```python
from build123d import *

# Parameters (mm, degrees)
BASE_FLANGE1_DEPTH                   = 3.175
EDGE_FLANGE1_DEPTH                   = 528.215976366
EDGE_FLANGE1_BEND_DEPTH              = 457.2
EDGE_FLANGE1_BEND_2_DEPTH            = 457.2
F_17_64_0_26563_DIAMETER_HOLE1_D     = 6.747002
F_17_64_0_26563_DIAMETER_HOLE1_DEPTH = 3.175
F_17_64_0_26563_DIAMETER_HOLE1_TIP   = 2.027003899
F_17_64_0_26563_DIAMETER_HOLE2_D     = 6.747002
F_17_64_0_26563_DIAMETER_HOLE2_DEPTH = 3.175
F_17_64_0_26563_DIAMETER_HOLE2_TIP   = 2.027003899
FILLET1_R                            = 3.175
F_17_64_0_26563_DIAMETER_HOLE3_D     = 6.747002
F_17_64_0_26563_DIAMETER_HOLE3_DEPTH = 3.175
F_17_64_0_26563_DIAMETER_HOLE3_TIP   = 2.027003899
F_17_64_0_26563_DIAMETER_HOLE4_D     = 6.747002


# Sheet-metal steps are written as plain solids
with BuildPart() as part:
    # Sketch1 → Base-Flange1 (new body)
    with BuildSketch(Plane(origin=(0, 0, 0), x_dir=(0, 0, -1), z_dir=(1, 0, 0))):
        Polygon((0, 12.7), (0, 469.9), (-11.934096284, 478.25634418), (-441.561562507, 321.884734651), (-443.092427829, 310.256658089), (-10.403230962, 7.284420742), align=None)
    extrude(amount=-BASE_FLANGE1_DEPTH)

    # Edge-Flange1 section (across the edge) → Edge-Flange1 (add)
    with BuildSketch(Plane(origin=(-3.175, 4.683613001, 12.224336148), x_dir=(-3.4914813388431334e-15, 0.819152044288993, -0.5735764363510446), z_dir=(0, 0.5735764363510446, 0.819152044288993))):
        with BuildLine():
            Line((-3.175, 3.175), (-3.175, 41.275))
            Line((-3.175, 41.275), (0, 41.275))
            Line((0, 41.275), (0, 3.175))
            ThreePointArc((0, 3.175), (0.92993597, 0.92993597), (3.175, 0))
            Line((3.175, 0), (3.175, -3.175))
            ThreePointArc((3.175, -3.175), (-1.315128061, -1.315128061), (-3.175, 3.175))
        make_face()
    extrude(amount=EDGE_FLANGE1_DEPTH)

    # Edge-Flange1 section 2 (across the edge) → Edge-Flange1 bend (add)
    with BuildSketch(Plane(origin=(-3.175, 469.9, -3.175), x_dir=(0, 0, 1), z_dir=(0, -1, 0))):
        with BuildLine():
            Line((-3.175, 3.175), (-3.175, 41.275))
            Line((-3.175, 41.275), (0, 41.275))
            Line((0, 41.275), (0, 3.175))
            ThreePointArc((0, 3.175), (0.92993597, 0.92993597), (3.175, 0))
            Line((3.175, 0), (3.175, -3.175))
            ThreePointArc((3.175, -3.175), (-1.315128061, -1.315128061), (-3.175, 3.175))
        make_face()
    extrude(amount=EDGE_FLANGE1_BEND_DEPTH)

    # Edge-Flange1 section 3 (across the edge) → Edge-Flange1 bend 2 (add)
    with BuildSketch(Plane(origin=(-3.175, 324.868258722, 442.647476462), x_dir=(-3.4914813388431334e-15, -0.9396926207859071, -0.3420201433256725), z_dir=(0, 0.3420201433256725, -0.9396926207859071))):
        with BuildLine():
            Line((-3.175, 3.175), (-3.175, 41.275))
            Line((-3.175, 41.275), (0, 41.275))
            Line((0, 41.275), (0, 3.175))
            ThreePointArc((0, 3.175), (0.92993597, 0.92993597), (3.175, 0))
            Line((3.175, 0), (3.175, -3.175))
            ThreePointArc((3.175, -3.175), (-1.315128061, -1.315128061), (-3.175, 3.175))
        make_face()
    extrude(amount=EDGE_FLANGE1_BEND_2_DEPTH)

    # 17/64 (0.26563) Diameter Hole1
    with Locations(Plane(origin=(0, 0, -6.35), x_dir=(-1, 0, 0), z_dir=(0, 0, -1))):
        with Locations((22.225, 390.525), (22.225, 31.75)):
            Hole(F_17_64_0_26563_DIAMETER_HOLE1_D / 2, depth=F_17_64_0_26563_DIAMETER_HOLE1_DEPTH)
            with Locations((0, 0, -(F_17_64_0_26563_DIAMETER_HOLE1_DEPTH + F_17_64_0_26563_DIAMETER_HOLE1_TIP / 2))):  # 118° drill point
                Cone(0, F_17_64_0_26563_DIAMETER_HOLE1_D / 2, F_17_64_0_26563_DIAMETER_HOLE1_TIP, mode=Mode.SUBTRACT)

    # 17/64 (0.26563) Diameter Hole2
    with Locations(Plane(origin=(0, 432.113572267, 157.276478127), x_dir=(1, 0, 0), z_dir=(3.4475760670445246e-15, 0.939692620785907, 0.3420201433256725))):
        with Locations((-22.225, 72.983921169), (-22.225, -285.791078831)):
            Hole(F_17_64_0_26563_DIAMETER_HOLE2_D / 2, depth=F_17_64_0_26563_DIAMETER_HOLE2_DEPTH)
            with Locations((0, 0, -(F_17_64_0_26563_DIAMETER_HOLE2_DEPTH + F_17_64_0_26563_DIAMETER_HOLE2_TIP / 2))):  # 118° drill point
                Cone(0, F_17_64_0_26563_DIAMETER_HOLE2_D / 2, F_17_64_0_26563_DIAMETER_HOLE2_TIP, mode=Mode.SUBTRACT)

    # Fillet1
    fillet1_edges = [part.edges().sort_by_distance(p)[0] for p in [
        (-44.45, 3.383209131, 13.134888741),
        (-44.45, 306.355446478, 445.824085607),
        (-44.45, 469.9, -4.7625),
        (-44.45, 12.7, -4.7625),
        (-44.45, 326.360020758, 443.19043344),
        (-44.45, 482.731630286, 13.562967217),
    ]]
    fillet(fillet1_edges, radius=FILLET1_R)

    # 17/64 (0.26563) Diameter Hole3
    with Locations(Plane(origin=(0, -5.201615481, 3.642210371), x_dir=(-1, 0, 0), z_dir=(2.9747797534781195e-15, -0.819152044288993, 0.5735764363510445))):
        with Locations((22.225, -48.207988183), (22.225, -200.607988183), (22.225, -353.007988183), (22.225, -505.407988183)):
            Hole(F_17_64_0_26563_DIAMETER_HOLE3_D / 2, depth=F_17_64_0_26563_DIAMETER_HOLE3_DEPTH)
            with Locations((0, 0, -(F_17_64_0_26563_DIAMETER_HOLE3_DEPTH + F_17_64_0_26563_DIAMETER_HOLE3_TIP / 2))):  # 118° drill point
                Cone(0, F_17_64_0_26563_DIAMETER_HOLE3_D / 2, F_17_64_0_26563_DIAMETER_HOLE3_TIP, mode=Mode.SUBTRACT)

    # 17/64 (0.26563) Diameter Hole4 (through all)
    with Locations(Plane(origin=(0, 0, 0), x_dir=(0, 0, -1), z_dir=(1, 0, 0))):
        with Locations((-410.363776349, 295.091728247), (-285.5250048, 207.678679347), (-160.68623325, 120.265630447), (-35.8474617, 32.852581547)):
            Hole(F_17_64_0_26563_DIAMETER_HOLE4_D / 2)


solid = part.part
```
Design review of the part built by this model. Coordinates are the model's own, in mm. A direction names the side the tool comes from. Give positions to 0.01 mm unless a question says otherwise; leave off trailing zeros. Write each loop counter-clockwise with the first axis right and the second up, starting at its lowest first coordinate (ties: lowest second). Pieces come first, ordered by that corner, then holes. Notation, with made-up numbers: (19.5, -33) - (64.5, -33) arc R18 cw to (64.5, -3) - close; hole circle Ø6 at (66, 30.5). An arc over 180 degrees is marked (long way). Return JSON: item names as keys, results as strings. Group by question number.
(1) To check wall thickness, follow probe 1 along X at (y, z) = (249, 337.5) (3 decimals); probe 2 along Z at (x, y) = (-42, 303) (3 decimals); probe 3 along Y at (x, z) = (-4.5, 135.5). State the ranges of each line that lie inside material, in increasing order.
(2) Insertion check: pin 1 (1.9 mm diameter, centred on x = -22.5, z = -2, fed in from +Y); pin 2 (8 mm diameter, centred on x = -5.5, z = 177.5, fed in from +Y); pin 3 (8 mm diameter, centred on y = 295.09, z = 410.36, fed in from +X); pin 4 (6 mm diameter, centred on x = -22.225, y = 31.75, fed in from +Z). Each pin has a flat end and moves straight along its axis. Give the tip position at first contact, or say it passes through.
(3) We need section A-A, the plane x = -35. Give the boundary of the cut face in (y, z) (3 decimals).
(4) Machinability: for faces 4 (the cylindrical face through (-4.13, 154.79, 225.02)), 5 (the flat face through (-26, 245, -3.175)), 6 (the flat face through (-25, 245, -6.35)), which of the approach directions +Z, -Z, +X, -X, +Y, -Y give a long, thin tool a straight path to every point of the face, cutting with its end or side? Answer none if there is none.
(5) Mouldability with a two-part tool opening along Z and no side actions: class faces 1 (the cylindrical face through (-4.13, 401.11, 230.53)), 2 (the cylindrical face through (-1.811, 153.012, 226.266)), 3 (the flat face through (0, 246, 175)) as +Z half, -Z half, draft (parallel to the pull), parting line (faces both ways), or undercut.
Reported:
{
 "1": {"probe 1": "x = -3.175 to 0", "probe 2": "z = -6.35 to -3.175, 438.264 to 443.8", "probe 3": "y = 87.46 to 91.73, 436.03 to 439.75"},
 "2": {"pin 1": "passes through", "pin 2": "stops at y = 426.19", "pin 3": "stops at x = 0", "pin 4": "stops at z = 60.7"},
 "3": {"outline": "(2.083, 14.045) - (4.684, 12.224) - (307.656, 444.914) - (305.055, 446.735) - close; (12.7, -6.35) - (469.9, -6.35) - (469.9, -3.175) - (12.7, -3.175) - close; (324.868, 442.647) - (481.24, 13.02) - (484.223, 14.106) - (327.852, 443.733) - close"},
 "4": {"face 4": "-X", "face 5": "-X, +Y, -Y", "face 6": "-Z, +X, -X, +Y, -Y"},
 "5": {"face 1": "undercut", "face 2": "+Z half", "face 3": "draft"}
}
